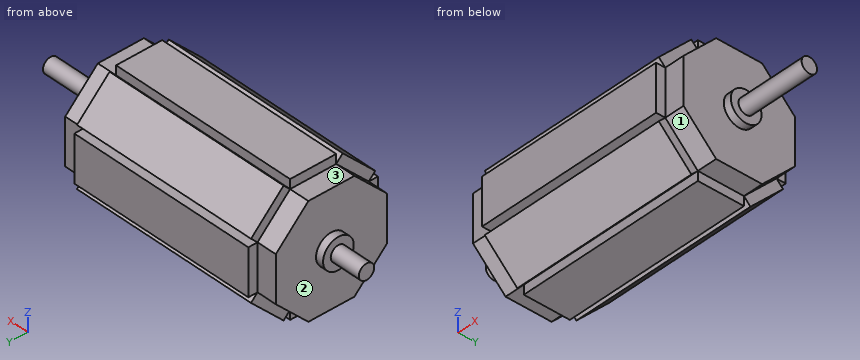
from build123d import *

# Parameters (mm, degrees)
EXTRUDE_1_DEPTH          = 30
SKETCH_4_R               = 1
EXTRUDE_2_DEPTH          = 10
SKETCH_5_R               = 2
EXTRUDE_3_DEPTH          = 1
EXTRUDE_START            = 5
SKETCH_6_R               = 1
EXTRUDE_4_DEPTH          = 5
EXTRUDE_START_2          = 1
SKETCH_7_R               = 2
EXTRUDE_5_DEPTH          = 1
SKETCH_8_W               = 24.796417242
SKETCH_8_H               = 6
EXTRUDE_6_DEPTH          = 1.2
PATTERN_CIRCULAR_1_COUNT = 8


with BuildPart() as part:
    # 草图1 → 凸台-拉伸1 (new body)
    with BuildSketch(Plane(origin=(0, 0, 0), x_dir=(0, 0, -1), z_dir=(1, 0, 0))):
        Polygon((7.242640687, -3), (7.242640687, 3), (3, 7.242640687), (-3, 7.242640687), (-7.242640687, 3), (-7.242640687, -3), (-3, -7.242640687), (3, -7.242640687), align=None)
    extrude(amount=EXTRUDE_1_DEPTH)

    # 草图4 → 凸台-拉伸2 (add)
    with BuildSketch(Plane(origin=(30, 0, 0), x_dir=(0, 0, -1), z_dir=(1, 0, 0))):
        Circle(SKETCH_4_R)
    extrude(amount=EXTRUDE_2_DEPTH)

    # 草图5 → 凸台-拉伸3 (add)
    with BuildSketch(Plane(origin=(30, 0, 0), x_dir=(0, 0, -1), z_dir=(1, 0, 0))):
        Circle(SKETCH_5_R)
    extrude(amount=EXTRUDE_3_DEPTH)

    # 草图6 → 凸台-拉伸4 (add)
    with BuildSketch(Plane.ZY.offset(EXTRUDE_START)):
        with Locations(Location((0, 0, 0), (0, 0, 180))):
            Circle(SKETCH_6_R)
    extrude(amount=-EXTRUDE_4_DEPTH)

    # 草图7 → 凸台-拉伸5 (add)
    with BuildSketch(Plane.ZY.offset(EXTRUDE_START_2)):
        with Locations(Location((0, 0, 0), (0, 0, 180))):
            Circle(SKETCH_7_R)
    extrude(amount=-EXTRUDE_5_DEPTH)

    # 草图8 → 凸台-拉伸6 (add)
    with BuildSketch(Plane(origin=(0, 7.242640687, 0), x_dir=(1, 0, 0), z_dir=(0, 1, 0))):
        with Locations((15, 0)):
            Rectangle(SKETCH_8_W, SKETCH_8_H)
    extrude_6 = extrude(amount=EXTRUDE_6_DEPTH)

    # 阵列(圆周)1: 凸台-拉伸6 ×8 about axis
    pattern_circular_1_axis = Axis((0, 0, 0), (1, 0, 0))
    for i in range(1, PATTERN_CIRCULAR_1_COUNT):
        add(extrude_6.rotate(pattern_circular_1_axis, i * 360 / PATTERN_CIRCULAR_1_COUNT))


solid = part.part
CAD build for the part. Positions are in the model's coordinates, mm. Face numbers are marked on the shaded views. A direction names the side the tool comes from. Round coordinates to 2 decimals unless told otherwise and drop trailing zeros. Loops run counter-clockwise (first coordinate to the right, second up) from the corner with the lowest first, then second, coordinate; pieces in that order, holes last. Notation, with made-up numbers: M -29,-31.75 L 24,-31.75 A27 cw 24,6.25 Z; hole C -24,31 d9. An arc over 180 degrees is marked long. One line per question, with ' | ' between items. Start each with the question number.
Item 1: Pin check, flat tips, straight feed: pin 1 Ø1.3 at (y, z) = (-7.5, 1) entering from +X; pin 2 Ø6 at (y, z) = (0, 6) entering from -X; pin 3 Ø1.3 at (x, z) = (1, -1.5) entering from -Y. Stop position of each tip, or through.
Item 2: Cut at A-A, the plane z = 0. Write the cut outline in (x, y).
Item 3: Wall check: line 1 (X direction, y = -2, z = 4.75); line 2 (Z direction, x = 27, y = -8); line 3 (X direction, y = -4.25, z = -7). Give the ranges that are in metal, low to high.
Item 4: Cut at D-D, the plane z = -2.5. Write the cut outline in (x, y).
Item 5: Which spindle directions (+Z, -Z, +X, -X, +Y, -Y) get a long thin tool onto all of the face, cutting with end or side? Do the marked faces 1, 2 and 3. Say none if no direction does.
Item 6: Cut at B-B, the plane x = 24.5. Write the cut outline in (y, z).
Responses:
1) pin 1: stops at x = 30 | pin 2: stops at x = 0 | pin 3: stops at y = -7.24
2) outline: M -5,-1 L -1,-1 L -1,-2 L 0,-2 L 0,-7.24 L 2.6,-7.24 L 2.6,-8.44 L 27.4,-8.44 L 27.4,-7.24 L 30,-7.24 L 30,-2 L 31,-2 L 31,-1 L 40,-1 L 40,1 L 31,1 L 31,2 L 30,2 L 30,7.24 L 27.4,7.24 L 27.4,8.44 L 2.6,8.44 L 2.6,7.24 L 0,7.24 L 0,2 L -1,2 L -1,1 L -5,1 Z
3) line 1: x = 0 to 30 | line 2: z = -3.94 to -3.76, -3 to 3, 3.76 to 3.94 | line 3: x = 2.6 to 27.4
4) outline: M 0,-7.24 L 2.6,-7.24 L 2.6,-8.44 L 27.4,-8.44 L 27.4,-7.24 L 30,-7.24 L 30,7.24 L 27.4,7.24 L 27.4,8.44 L 2.6,8.44 L 2.6,7.24 L 0,7.24 Z
5) face 1: -Z, +X, -Y | face 2: -X | face 3: +Z, -X, +Y, -Y
6) outline: M -8.44,-3 L -7.24,-3 L -8.09,-3.85 L -3.85,-8.09 L -3,-7.24 L -3,-8.44 L 3,-8.44 L 3,-7.24 L 3.85,-8.09 L 8.09,-3.85 L 7.24,-3 L 8.44,-3 L 8.44,3 L 7.24,3 L 8.09,3.85 L 3.85,8.09 L 3,7.24 L 3,8.44 L -3,8.44 L -3,7.24 L -3.85,8.09 L -8.09,3.85 L -7.24,3 L -8.44,3 Z
